Read the model definition and answer for the solid it produces. Units are mm, in the model's axes. A direction names the side the tool comes from. Give positions to 0.01 mm unless a question says otherwise; leave off trailing zeros. Loops run counter-clockwise (first coordinate to the right, second up) from the corner with the lowest first, then second, coordinate; pieces in that order, holes last. Notation, with made-up numbers: M 32,55.25 L 65,55.25 A26 ccw 65,79.25 Z; hole C -25,70 d4. An arc over 180 degrees is marked long. Return JSON: item names as keys, results as strings. Group by question number.
```python
from build123d import *

# Parameters (mm, degrees)
SKETCH1_W               = 101.6
SKETCH1_H               = 50.8
BOSS_EXTRUDE1_DEPTH     = 50.8
BOSS_EXTRUDE2_DEPTH     = 101.6
CUT_EXTRUDE1_DEPTH      = 101.6
SHELL1_T                = -2.54
SKETCH4_W               = 101.6
SKETCH4_H               = 2.54
BOSS_EXTRUDE3_DEPTH     = 12.7
CUT_EXTRUDE2_DEPTH      = 2.54
LPATTERN1_COUNT         = 11
LPATTERN1_PITCH         = 9.652
CUT_EXTRUDE3_DEPTH      = 109.22
CUT_EXTRUDE3_DEPTH_BACK = 5.08
SKETCH6_W               = 39.172348931
SKETCH6_H               = 64.321849683


with BuildPart() as part:
    # Sketch1 → Boss-Extrude1 (new body)
    with BuildSketch(Plane.XY):
        with Locations((50.8, 25.4)):
            Rectangle(SKETCH1_W, SKETCH1_H)
    extrude(amount=-BOSS_EXTRUDE1_DEPTH)

    # Sketch2 → Boss-Extrude2 (add)
    with BuildSketch(Plane.ZY):
        with BuildLine():
            Line((-50.8, 50.8), (-50.8, 0))
            ThreePointArc((-50.8, 0), (-76.2, 25.4), (-50.8, 50.8))
        make_face()
    extrude(amount=-BOSS_EXTRUDE2_DEPTH)

    # Sketch3 → Cut-Extrude1 (cut)
    with BuildSketch(Plane.ZY):
        Polygon((0, 0), (-25.4, 50.8), (0, 50.8), align=None)
    extrude(amount=-CUT_EXTRUDE1_DEPTH, mode=Mode.SUBTRACT)

    # Shell1
    shell1_openings = [part.faces().sort_by_distance(p)[0] for p in [
        (50.8, 25.4, -12.7),
    ]]
    offset(amount=SHELL1_T, openings=shell1_openings, kind=Kind.INTERSECTION)

    # Sketch4 → Boss-Extrude3 (add)
    with BuildSketch(Plane.XY.offset(-2.54)):
        with Locations((50.8, 1.27)):
            Rectangle(SKETCH4_W, SKETCH4_H)
    extrude(amount=BOSS_EXTRUDE3_DEPTH)

    # Sketch5 → Cut-Extrude2 (cut)
    with BuildSketch(Plane(origin=(0, 2.54, 0), x_dir=(1, 0, 0), z_dir=(0, 1, 0))):
        Polygon((0, 0), (4.208409794, -10.16), (0, -10.16), align=None)
        Polygon((5.478409794, -10.16), (9.686819587, 0), (9.686819587, -10.16), align=None)
    cut_extrude2 = extrude(amount=-CUT_EXTRUDE2_DEPTH, mode=Mode.SUBTRACT)

    # LPattern1: Cut-Extrude2 ×11
    with Locations(*[(i * LPATTERN1_PITCH, 0, 0) for i in range(1, LPATTERN1_COUNT)]):
        add(cut_extrude2, mode=Mode.SUBTRACT)

    # Sketch6 → Cut-Extrude3 (cut, two sides: drawn at the far end of the back side and taken through both)
    with BuildSketch(Plane.ZY.offset(-99.06).offset(-CUT_EXTRUDE3_DEPTH_BACK)):
        with Locations((-71.087050569, 22.645845649)):
            Rectangle(SKETCH6_W, SKETCH6_H)
    extrude(amount=CUT_EXTRUDE3_DEPTH + CUT_EXTRUDE3_DEPTH_BACK, mode=Mode.SUBTRACT)


solid = part.part
```
1. A flat-ended cylindrical pin translates along its axis: P1, Ø1.5, axis at x = 89.5, z = -16, coming from the +Y side. Find the tip coordinate at first contact, or state that the pin passes through.
2. Find section A-A (y = 8). Write down the section's boundary in (x, z), and give its area (3 significant figures).
3. The mould has two halves that part along X. Classify faces 1 (the flat face through (65.45, 1.29, 5.19)), 2 (the flat face through (0, 25, -32)), 3 (the flat face through (51, 50, -25)), 4 (the flat face through (60.004, 1.288, 5.051)): +X half, -X half, draft (parallel to the pull), parting line (faces both ways), or undercut.
4. For faces 5 (the flat face through (2.54, 26, -32)), 6 (the flat face through (50, 50.8, -38)), 7 (the flat face through (17.19, 1.29, 5.19)), determine the directions among +Z, -Z, +X, -X, +Y, -Y from which every point of the face is accessible in a straight line to the end or side of a thin tool.
5. Straight lines are drawn through the part: line 1 along X through (y, z) = (7.5, -15.5); line 2 along Y through (x, z) = (76.5, -48.5); line 3 along Y through (x, z) = (9.5, -3.5). For each, find the intervals that lie inside material, in ascending order.
6. Find section B-B (z = -46). Write down the section's boundary in (x, y).
7. Find section C-C (x = 79.5). Write down the section's boundary in (y, z).
8. Find section D-D (y = 34.5). Write down the section's boundary in (x, z), and give its area (3 significant figures).
Result:
{
 "1": {"P1": "stops at y = 2.54"},
 "2": {"outline": "M 0,-51.5 L 2.54,-51.5 L 2.54,-4 L 0,-4 Z; M 99.06,-51.5 L 101.6,-51.5 L 101.6,-4 L 99.06,-4 Z", "area": "241 mm2"},
 "3": {"face 1": "undercut", "face 2": "-X half", "face 3": "draft", "face 4": "undercut"},
 "4": {"face 5": "+Z, -Z", "face 6": "+Z, -Z, +X, -X, +Y", "face 7": "+Z, +Y, -Y"},
 "5": {"line 1": "x = 0 to 2.54, 99.06 to 101.6", "line 2": "y = 0 to 2.54, 48.26 to 50.8", "line 3": "y = 0 to 2.54"},
 "6": {"outline": "M 0,0 L 101.6,0 L 101.6,50.8 L 0,50.8 Z; hole M 2.54,2.54 L 99.06,2.54 L 99.06,48.26 L 2.54,48.26 Z"},
 "7": {"outline": "M 0,-50.8 A25.4 ccw 0.01,-51.5 L 2.55,-51.5 A22.86 cw 2.54,-50.8 L 2.54,5.51 L 0,5.51 Z; M 48.25,-51.5 L 50.79,-51.5 A25.4 ccw 50.8,-50.8 L 50.8,-25.4 L 48.26,-24.13 L 48.26,-50.8 A22.86 cw Z"},
 "8": {"outline": "M 0,-51.5 L 2.54,-51.5 L 2.54,-17.25 L 0,-17.25 Z; M 99.06,-51.5 L 101.6,-51.5 L 101.6,-17.25 L 99.06,-17.25 Z", "area": "174 mm2"}
}
